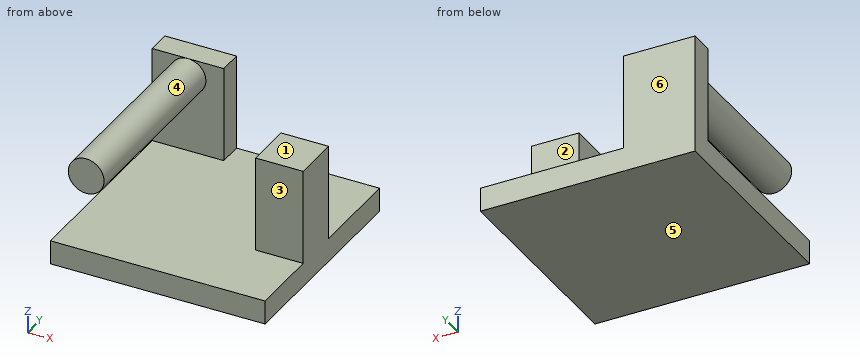
from build123d import *

# Parameters (mm, degrees)
F0_W     = 114.3
F0_H     = 114.3
F1_DEPTH = 12.7
F2_W     = 38.1
F2_H     = 12.7
F3_DEPTH = 50.8
F5_DEPTH = 101.6
F7_DEPTH = 50.8


with BuildPart() as f1:
    # F0 (on Top) → F1 (new body)
    with BuildSketch(Plane.XY):
        with Locations((57.15, -57.15)):
            Rectangle(F0_W, F0_H)
    extrude(amount=F1_DEPTH)

    # F2 (on face) → F3 (join)
    with BuildSketch(Plane.XY.offset(12.7)):
        with Locations((19.05, -6.35)):
            Rectangle(F2_W, F2_H)
    extrude(amount=F3_DEPTH)

    # F4 (on face) → F5 (join, through all)
    with BuildSketch(Plane.XZ.offset(12.7)):
        with BuildLine():
            Line((9.525, 53.975), (28.575, 53.975))
            ThreePointArc((28.575, 53.975), (19.05, 63.5), (9.525, 53.975))
        make_face()
        with BuildLine():
            ThreePointArc((9.525, 53.975), (19.05, 44.45), (28.575, 53.975))
            Line((28.575, 53.975), (9.525, 53.975))
        make_face()
    extrude(amount=F5_DEPTH)

    # F6 (on face) → F7 (join, through all)
    with BuildSketch(Plane.XY.offset(12.7)):
        Polygon((114.3, -76.2), (114.3, -50.8), (88.9, -50.8), (88.9, -63.5), (88.9, -76.2), align=None)
    extrude(amount=F7_DEPTH)


solid = f1.part
Design review of the part built by this model. Coordinates are the model's own, in mm. Face numbers are marked on the shaded views. A direction names the side the tool comes from. Give positions to 0.01 mm unless a question says otherwise; leave off trailing zeros. Write each loop counter-clockwise with the first axis right and the second up, starting at its lowest first coordinate (ties: lowest second). Pieces come first, ordered by that corner, then holes. Notation, with made-up numbers: M 16,0 L 27,0 A20 cw 27,27 Z; hole C 66,51 d5. An arc over 180 degrees is marked long. Return JSON: item names as keys, results as strings. Group by question number.
Item 1: Wall thickness on line 1 along X through (y, z) = (-12, 15.5); line 2 along Z through (x, y) = (95.5, -6); line 3 along Z through (x, y) = (13, -27): over which ranges is each line inside the solid? List them lowest first.
Item 2: The part is to be moulded in two halves that separate along Z. For the marked faces 4, 5 and 6, say which applies: pulls with the +Z half, pulls with the -Z half, needs draft (parallel to the pull), parting line crosses it, or undercut.
Item 3: Clearance check with flat-ended pins moving along their axes: pin 1 Ø5 at (y, z) = (-23, 43) entering from +X; pin 2 Ø1 at (x, y) = (86.5, -85) entering from +Z; pin 3 Ø12 at (y, z) = (-96.5, 42.5) entering from +X. State where each tip first meets the part, or that it passes through.
Item 4: Take a section at D-D (z = 55.5). Give the boundary of the cut face in (x, y), plus the area to 3 significant figures.
Item 5: Take a section at B-B (x = 30). Give the boundary of the cut face in (y, z), plus the area to 3 significant figures.
Item 6: Take a section at C-C (y = -48.5). Give the boundary of the cut face in (x, z) (3 decimals), plus the area to 3 significant figures.
Item 7: Take a section at A-A (z = 17). Give the boundary of the cut face in (x, y).
Item 8: Tool access review of the marked faces 1, 2 and 3: name each direction out of +Z, -Z, +X, -X, +Y, -Y from which nothing blocks a thin tool from reaching the whole face with its end or side.
Return value:
{
 "1": {"line 1": "x = 0 to 38.1", "line 2": "z = 0 to 12.7", "line 3": "z = 0 to 12.7, 46.62 to 61.33"},
 "2": {"face 4": "undercut", "face 5": "pulls with the -Z half", "face 6": "needs draft"},
 "3": {"pin 1": "stops at x = 23.4", "pin 2": "stops at z = 12.7", "pin 3": "stops at x = 26.84"},
 "4": {"outline": "M 0,-12.7 L 9.65,-12.7 L 9.65,-114.3 L 28.45,-114.3 L 28.45,-12.7 L 38.1,-12.7 L 38.1,0 L 0,0 Z; M 88.9,-76.2 L 114.3,-76.2 L 114.3,-50.8 L 88.9,-50.8 Z", "area": "3,040 mm2"},
 "5": {"outline": "M -114.3,0 L 0,0 L 0,63.5 L -12.7,63.5 L -12.7,12.7 L -114.3,12.7 Z", "area": "2,100 mm2"},
 "6": {"outline": "M 0,0 L 114.3,0 L 114.3,12.7 L 0,12.7 Z; C 19.05,53.975 d19.05", "area": "1,740 mm2"},
 "7": {"outline": "M 0,-12.7 L 38.1,-12.7 L 38.1,0 L 0,0 Z; M 88.9,-76.2 L 114.3,-76.2 L 114.3,-50.8 L 88.9,-50.8 Z"},
 "8": {"face 1": "+Z, +X, -X, +Y, -Y", "face 2": "+Z, +X, +Y", "face 3": "+Z, +X, -Y"}
}
